from build123d import *

# Parameters (mm, degrees)
F1_DEPTH = 228.6
F2_R     = 1
F3_W     = 25
F3_H     = 2.1
F4_DEPTH = 20
F5_W     = 12
F5_H     = 1
F6_DEPTH = 8


with BuildPart() as f1:
    # F0 (on Front) → F1 (new body)
    with BuildSketch(Plane.XZ):
        Polygon((183.579294, 53.486018), (83.579294, 53.486018), (-16.420706, 53.486018), (-38.13115, 53.486018), (-170.113422, -175.113982), (-140.784028, -175.113982), (-23.466453, 28.086018), (83.579294, 28.086018), (190.625042, 28.086018), (307.942616, -175.113982), (337.27201, -175.113982), (205.289739, 53.486018), align=None)
        with BuildLine():
            Line((-38.13115, 53.486018), (-16.420706, 53.486018))
            Line((-16.420706, 53.486018), (-16.420706, 58.486018))
            ThreePointArc((-16.420706, 58.486018), (-25.888059, 55.488385), (-35.470706, 58.094042))
            Line((-35.470706, 58.094042), (-38.13115, 53.486018))
        make_face()
        with BuildLine():
            Line((183.579294, 58.486018), (183.579294, 53.486018))
            Line((183.579294, 53.486018), (205.289739, 53.486018))
            Line((205.289739, 53.486018), (202.629294, 58.094042))
            ThreePointArc((202.629294, 58.094042), (193.046647, 55.488385), (183.579294, 58.486018))
        make_face()
    extrude(amount=F1_DEPTH)

    # F2
    f2_edges = [f1.edges().sort_by_distance(p)[0] for p in [
        (-35.470706, -114.3, 58.094042),
        (-16.420706, -114.3, 58.486018),
        (183.579294, -114.3, 58.486018),
        (202.629294, -114.3, 58.094042),
        (-170.113422, -114.3, -175.113982),
        (-140.784028, -114.3, -175.113982),
        (307.942616, -114.3, -175.113982),
        (337.27201, -114.3, -175.113982),
    ]]
    fillet(f2_edges, radius=F2_R)

    # F3 (on face) → F4 (cut)
    with BuildSketch(Plane.XZ.offset(228.6)):
        with Locations((170.792693, 39.736018)):
            Rectangle(F3_W, F3_H)
        with Locations((139.442693, 39.736018)):
            Rectangle(F3_W, F3_H)
        with Locations((108.092693, 39.736018)):
            Rectangle(F3_W, F3_H)
    extrude(amount=-F4_DEPTH, mode=Mode.SUBTRACT)

    # F5 (on face) → F6 (cut)
    with BuildSketch(Plane.XZ.offset(228.6)):
        with Locations((83.242693, 39.186018)):
            Rectangle(F5_W, F5_H)
        with Locations((64.892693, 39.186018)):
            Rectangle(F5_W, F5_H)
        with Locations((46.542693, 39.186018)):
            Rectangle(F5_W, F5_H)
    extrude(amount=-F6_DEPTH, mode=Mode.SUBTRACT)


solid = f1.part
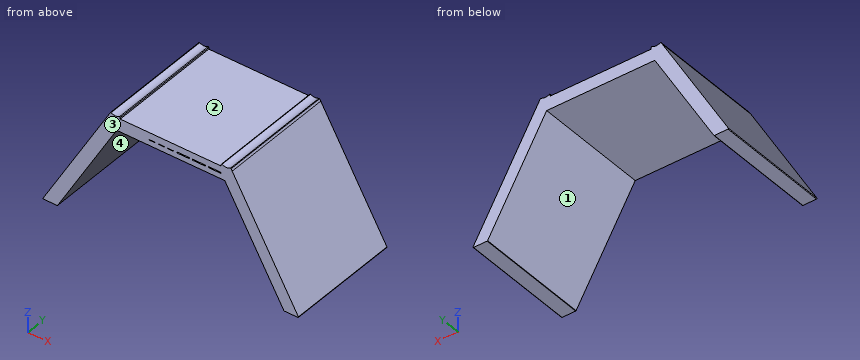
Verification items for the finished model (mm, model axes). Face numbers are marked on the shaded views. A direction names the side the tool comes from. Round coordinates to 2 decimals unless told otherwise and drop trailing zeros. Write each loop counter-clockwise with the first axis right and the second up, starting at its lowest first coordinate (ties: lowest second). Pieces come first, ordered by that corner, then holes.
(1) Section check A-A (z = -110). Enter the section's corners in (x, y).
Returned:
outline: (-132.52, -228.6) - (-103.19, -228.6) - (-103.19, 0) - (-132.52, 0) - close; (270.35, -228.6) - (299.68, -228.6) - (299.68, 0) - (270.35, 0) - close
(2) Section check B-B (y = -39.5). Enter the section's corners in (x, z).
Returned:
outline: (-169.25, -173.61) arc R1 ccw to (-168.38, -175.11) - (-141.36, -175.11) arc R1 ccw to (-140.5, -174.61) - (-23.47, 28.09) - (190.63, 28.09) - (307.65, -174.61) arc R1 ccw to (308.52, -175.11) - (335.54, -175.11) arc R1 ccw to (336.41, -173.61) - (205.29, 53.49) - (203.13, 57.23) arc R1 ccw to (201.79, 57.61) arc R17.6 cw to (185.05, 57.59) arc R1 ccw to (183.58, 56.71) - (183.58, 53.49) - (-16.42, 53.49) - (-16.42, 56.71) arc R1 ccw to (-17.9, 57.59) arc R17.6 cw to (-34.63, 57.61) arc R1 ccw to (-35.97, 57.23) - close
(3) Depth check by flat-ended pin: pin 1 Ø3.5 at (y, z) = (-64, 54.5) entering from -X; pin 2 Ø8 at (x, y) = (102.5, -79.5) entering from -Z; pin 3 Ø2.5 at (x, y) = (66.5, -224) entering from +Z; pin 4 Ø10 at (x, z) = (240.5, -34.5) entering from +Y. Enter the tip coordinate at first touch or a pass-through.
Returned:
pin 1: stops at x = -38.56
pin 2: stops at z = 28.09
pin 3: stops at z = 53.49
pin 4: stops at y = 0
(4) Material ranges on line 1 (Z direction, x = 68, y = -165.5); line 2 (X direction, y = -196, z = -104); line 3 (X direction, y = -21.5, z = -69.5), recorded low to high.
Returned:
line 1: z = 28.09 to 53.49
line 2: x = -129.06 to -99.73, 266.88 to 296.21
line 3: x = -109.14 to -79.81, 246.97 to 276.3
(5) Section check D-D (z = 33.5). Enter the section's corners in (x, y), plus the area to 3 significant figures.
Returned:
outline: (-49.67, -228.6) - (216.83, -228.6) - (216.83, 0) - (-49.67, 0) - close
area: 60,900 mm2
(6) Access from +Z, -Z, +X, -X, +Y, -Y to the whole of each face (thin tool, end or side, straight path). Record for the marked faces 1 and 2.
Returned:
face 1: -Z, +Y, -Y
face 2: +Z, +Y, -Y
(7) Mould release check, pull along X, two halves, no side actions. Record for the marked faces 3 and 4: pulls with the +X half, pulls with the -X half, needs draft (parallel to the pull), parting line crosses it, or undercut.
Returned:
face 3: needs draft
face 4: undercut
(8) Section check C-C (x = -102). Enter the section's corners in (y, z).
Returned:
outline: (-228.6, -107.94) - (0, -107.94) - (0, -57.14) - (-228.6, -57.14) - close
